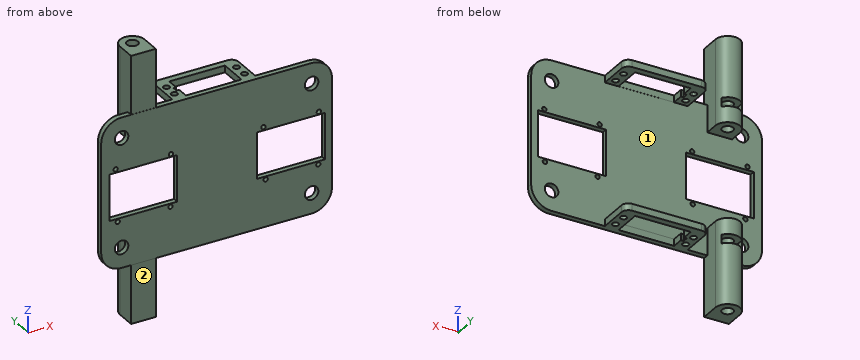
Autodesk Inventor part; units mm, degrees
ref_plane "Work Plane1" through (0, 0, 0) normal (0, 0, -1) x (-1, 0, 0)
ref_plane "YZ Plane" through (0, 0, 0) normal (1, 0, 0) x (0, 1, 0)
ref_plane "XZ Plane" through (0, 0, 0) normal (0, 1, 0) x (-1, 0, 0)
sketch "Sketch1" plane through (0, 0, 0) normal (0, 0, 1) x (1, 0, 0)
  line L0 (-20.5, 0.0342) -> (20.5, 0.0342)
  line L1 (20.5, 0.0342) -> (20.5, 21.0342)
  line L2 (20.5, 21.0342) -> (-20.5, 21.0342)
  line L3 (-20.5, 21.0342) -> (-20.5, 0.0342)
  line L4 (0, -10.9658) -> (0, 38.0342)
  line L5 (20.5, 0.0342) -> (27.5, 0.0342)
  line L6 (20.5, 18.3469) -> (20.5, 0.0342)
  line L7 (20.5, 1.1342) -> (27.5, 1.1342)
  line L8 (27.5, 1.1342) -> (27.5, 19.9342)
  line L9 (27.5, 19.9342) -> (20.5, 19.9342)
  line L10 (20.5, 19.9342) -> (20.5, 1.1342)
  circle A0 centre (25.8, 15.5342) radius 2.3
  circle A1 centre (25.8, 5.5342) radius 2.3
  line L11 (-20.5, 0.0342) -> (-27.5, 0.0342)
  line L12 (-20.5, 1.1342) -> (-27.5, 1.1342)
  line L13 (-27.5, 19.9342) -> (-20.5, 19.9342)
  circle A2 centre (-25.8, 15.5342) radius 2.3
  circle A3 centre (-25.8, 5.5342) radius 2.3
  line L14 (-30.5, 0.0342) -> (-30.5, 31.0342)
  line L15 (30.5, 31.0342) -> (30.5, 0.0342)
  line L16 (-30.5, 26.0342) -> (30.5, 26.0342)
  line L17 (-27.5, 1.1342) -> (-27.5, 13.985)
  line L18 (-27.5, 17.0834) -> (-27.5, 19.9342)
  line L19 (-20.5, 8.5342) -> (-22.5, 8.5342)
  line L20 (-22.5, 8.5342) -> (-22.5, 12.5342)
  line L21 (-22.5, 12.5342) -> (-20.5, 12.5342)
  line L22 (-20.5, 9.5596) -> (-20.5, 7.5596)
  line L23 (-21.9602, 10.5342) -> (-18.6691, 10.5342)
  line L24 (-30.5, 0.0342) -> (-26.5, 0.0342)
  line L25 (-30.5, 0.0342) -> (30.5, 0.0342)
  line L26 (30.5, 0.0342) -> (30.5, -3.9658)
  line L27 (30.5, -3.9658) -> (-30.5, -3.9658)
  line L28 (-30.5, -3.9658) -> (-30.5, 0.0342)
  point P0 (0, 0)
  point P1 (30.5, 0.0342)
  dimension "d0" = 41
  dimension "d4" = 7
  dimension "d5" = 18.8
  dimension "d6" = 1.1
  dimension "d7" = 21
  dimension "d8" = 4.6
  dimension "d9" = 4.6
  dimension "d10" = 5.3
  dimension "d11" = 10
  dimension "d12" = 4.4
  dimension "d13" = 4.4
  dimension "d14" = 10
  dimension "d15" = 5
  dimension "d16" = 2
  dimension "d17" = 4
  dimension "d19" = 4
extrude "Extrusion1" add sketch "Sketch1" along normal blind 5 contours L11 L24 L14 L16 L4 L2 L3 L13 L18 A2 L17 A3 L12 | L0 L4 L27 L28 L24 L11 | L0 L5 L25 L26 L27 L4 | L12 L17 A3 A2 L18 L13 L3 L21 L20 L19 | L1 L7 L8 A1 A0 L9 L2 L4 L16 L15 L25 L5 | L1 L9 L8 A0 A1 L7
sketch "Sketch2" plane through (0, 0, 5) normal (0, 0, 1) x (1, 0, 0)
  line L0 (20.5, 0.0342) -> (-20.5, 0.0342)
  line L1 (20.5, 0.0342) -> (12.9, 0.0342)
  line L2 (12.9, 0.0342) -> (12.9, 10.0342)
  line L3 (12.9, 10.0342) -> (-54.1, 10.0342)
  circle A0 centre (-54.1, 10.0342) radius 4.1
  circle A1 centre (-54.1, 10.0342) radius 9.1
  line L4 (-63.2, 10.0342) -> (-63.2, 0.0342)
  line L5 (-45, 10.0342) -> (-45, 0.0342)
  line L6 (-63.2, 0.0342) -> (-45, 0.0342)
  line L7 (-63.2, 0.0342) -> (-45, 0.0342)
  line L8 (-45, 0.0342) -> (-45, -3.9658)
  line L9 (-45, -3.9658) -> (-63.2, -3.9658)
  line L10 (-63.2, -3.9658) -> (-63.2, 0.0342)
  point P0 (0, 0)
  dimension "d22" = 7.6
  dimension "d23" = 10
  dimension "d24" = 67
  dimension "d25" = 8.2
  dimension "d26" = 5
  dimension "d29" = 4
extrude "Extrusion2" add sketch "Sketch2" along normal blind 43
sketch "Sketch5" plane through (0, 0, 0) normal (0, 1, 0) x (-1, 0, 0)
  line L0 (-20.5, 0) -> (-20.5, 5)
  line L1 (20.5, 0) -> (20.5, 5)
  line L2 (14.7818, 0) -> (56.1092, 0)
  line L3 (56.1092, 0) -> (56.1092, -28.5)
  line L4 (56.1092, -28.5) -> (14.7818, -28.5)
  line L5 (14.7818, -28.5) -> (14.7818, 0)
  line L6 (17.451, -24.4449) -> (17.451, -8.948) construction
  line L7 (17.451, -8.948) -> (25.6459, -8.948) construction
  line L8 (25.6459, -8.948) -> (25.6459, -24.4449) construction
  line L9 (25.6459, -24.4449) -> (17.451, -24.4449) construction
  line L10 (-84.7718, 5) -> (85.2282, 5)
  line L11 (85.2282, 5) -> (85.2282, -50)
  line L12 (85.2282, -50) -> (-84.7718, -50)
  line L13 (-84.7718, -50) -> (-84.7718, 5)
  point P0 (0, 0)
  point P1 (30.5, 5)
  dimension "d30" = 28.5
  dimension "d49" = 55
  dimension "d60" = 170
sketch "Sketch7" plane through (0, 0, 0) normal (0, 1, 0) x (-1, 0, 0)
  point P0 (0, 0)
sketch "Sketch8" plane through (0, 0, 5) normal (0, 0, -1) x (-1, 0, 0)
  line L0 (63.2, 10.0342) -> (63.2, -3.9658)
  arc A0 (63.2, 10.0342) -> (45, 10.0342) centre (54.1, 10.0342) ccw
  line L1 (45, -3.9658) -> (45, 10.0342)
  line L2 (63.2, -3.9658) -> (45, -3.9658)
  circle A1 centre (54.1, 10.0342) radius 4.1
  line L3 (63.2, 10.0342) -> (63.2, -3.9658)
  line L4 (63.2, 0) -> (45, 0)
  point P0 (0, 0)
extrude "Extrusion4" add sketch "Sketch8" along normal blind 20 contours L0 L4 L1 A0
extrude "Extrusion5" add sketch "Sketch5" against normal blind 4 contours L10 L11 L12 L13 | L2 L3 L4 L5
ref_plane "Work Plane1" through (0, 0, 0) normal (0, 0, -1) x (-1, 0, 0)
sketch "Sketch9" plane through (0, 0, 0) normal (0, 0, -1) x (-1, 0, 0)
  line L0 (45, 10.0342) -> (45, 0)
  line L1 (45, 0) -> (63.2, 0)
  line L2 (63.2, 0) -> (63.2, 10.0342)
  arc A0 (63.2, 10.0342) -> (45, 10.0342) centre (54.1, 10.0342) ccw
  circle A1 centre (54.1, 10.0342) radius 4.1
  line L3 (61.6056, 10.0342) -> (57.8528, 3.5342)
  line L4 (57.8528, 3.5342) -> (50.3472, 3.5342)
  line L5 (50.3472, 3.5342) -> (46.5944, 10.0342)
  line L6 (46.5944, 10.0342) -> (50.3472, 16.5342)
  line L7 (50.3472, 16.5342) -> (57.8528, 16.5342)
  line L8 (57.8528, 16.5342) -> (61.6056, 10.0342)
  line L9 (46.5944, 10.0342) -> (46.5944, 15.1797)
  arc A2 (63.2, 10.0342) -> (45, 10.0342) centre (54.1, 10.0342) ccw
  line L10 (61.6056, 10.0342) -> (61.6056, 15.1797)
  point P0 (0, 0)
  dimension "d43" = 13
extrude "Extrusion6" cut sketch "Sketch9" along normal mid plane 6.5 contours A0 L10 L8 L7 L6 L9 | L6 L7 L8 L3 L4 L5
fillet "Fillet2" radius 15 2 edges at (84.7718, -2, 5) (-85.2282, -2, 5)
fillet "Fillet3" radius 5 2 edges at (30.5, 26.0342, 2.5) (-30.5, 26.0342, 2.5)
sketch "Sketch10" plane through (0, 0, 0) normal (0, 1, 0) x (1, 0, 0)
  arc A0 (-85.2282, 10) -> (-70.2282, -5) centre (-70.2282, 10) ccw
  line L0 (-63.2, -5) -> (-63.2, 15)
  line L1 (-45, 15) -> (-63.2, 15)
  line L2 (-45, -5) -> (-45, 15)
  line L3 (-45, -5) -> (-30.5, -5)
  line L4 (-30.5, 0) -> (-30.5, -5)
  line L5 (30.5, 0) -> (-30.5, 0)
  line L6 (30.5, -5) -> (30.5, 0)
  line L7 (30.5, -5) -> (69.7718, -5)
  arc A1 (69.7718, -5) -> (84.7718, 10) centre (69.7718, 10) ccw
  line L8 (84.7718, 10) -> (84.7718, 50)
  line L9 (84.7718, 50) -> (-85.2282, 50)
  line L10 (-85.2282, 50) -> (-85.2282, 10)
  line L11 (-70.2282, -5) -> (-63.2, -5)
  point P0 (0, 0)
hole "Hole1" at (-70.2282, 0, -10) at (69.7718, 0, -10) direction (0, -1, 0) diameter 10 depth 4
mirror "Mirror4" about plane through (-85.2282, 0, -50) normal (0, 0, -1) of "Extrusion1", "Extrusion2", "Extrusion4", "Extrusion5", "Extrusion6", "Fillet2", "Fillet3", "Hole1"
sketch "Sketch11" plane through (0, 0, 0) normal (0, 1, 0) x (1, 0, 0)
  circle A0 centre (69.7718, 90) radius 5
  circle A1 centre (69.7718, 10) radius 5
  arc A2 (-70.2282, 105) -> (-85.2282, 90) centre (-70.2282, 90) ccw
  line L0 (-85.2282, 90) -> (-85.2282, 10)
  arc A3 (-85.2282, 10) -> (-70.2282, -5) centre (-70.2282, 10) ccw
  line L1 (-63.2, -5) -> (-63.2, 15)
  line L2 (-45, 15) -> (-63.2, 15)
  line L3 (-45, -5) -> (-45, 15)
  line L4 (-45, -5) -> (-30.5, -5)
  line L5 (-30.5, 0) -> (-30.5, -5)
  line L6 (30.5, 0) -> (-30.5, 0)
  line L7 (30.5, -5) -> (30.5, 0)
  line L8 (30.5, -5) -> (69.7718, -5)
  arc A4 (69.7718, -5) -> (84.7718, 10) centre (69.7718, 10) ccw
  line L9 (84.7718, 10) -> (84.7718, 90)
  arc A5 (84.7718, 90) -> (69.7718, 105) centre (69.7718, 90) ccw
  line L10 (30.5, 105) -> (69.7718, 105)
  line L11 (30.5, 105) -> (30.5, 100)
  line L12 (30.5, 100) -> (-30.5, 100)
  line L13 (-30.5, 100) -> (-30.5, 105)
  line L14 (-45, 105) -> (-30.5, 105)
  line L15 (-45, 105) -> (-45, 85)
  line L16 (-45, 85) -> (-63.2, 85)
  line L17 (-63.2, 105) -> (-63.2, 85)
  line L18 (20.5, 100) -> (-20.5, 100)
  line L19 (20.5, 100) -> (20.5, 105)
  line L20 (20.5, 105) -> (-20.5, 105)
  line L21 (-20.5, 100) -> (-20.5, 105)
  line L22 (-20.5, 100) -> (20.5, 100)
  line L23 (20.5, 100) -> (20.5, 71.5)
  line L24 (20.5, 71.5) -> (-20.5, 71.5)
  line L25 (-20.5, 71.5) -> (-20.5, 100)
  line L26 (74.1747, 78.4479) -> (24.1747, 78.4479)
  line L27 (24.1747, 78.4479) -> (24.1747, 28.4479)
  line L28 (24.1747, 28.4479) -> (74.1747, 28.4479)
  line L29 (74.1747, 28.4479) -> (74.1747, 78.4479)
  line L30 (0, 73.183) -> (0, 43.8378)
  line L31 (-78.2096, 79.1815) -> (-28.2096, 79.1815)
  line L32 (-28.2096, 79.1815) -> (-28.2096, 29.1815)
  line L33 (-28.2096, 29.1815) -> (-78.2096, 29.1815)
  line L34 (-78.2096, 29.1815) -> (-78.2096, 79.1815)
  circle A6 centre (-70.2282, 90) radius 5
  line L35 (-70.2282, 105) -> (-63.2, 105)
  line L36 (-70.2282, -5) -> (-63.2, -5)
  circle A7 centre (-70.2282, 10) radius 5
  point P0 (0, 0)
  dimension "d57" = 28.5
  dimension "d58" = 50
  dimension "d59" = 50
sketch "Sketch12" plane through (0, 0, 0) normal (0, 1, 0) x (1, 0, 0)
  line L0 (-79.2036, 26.0949) -> (-29.2036, 26.0949)
  line L1 (-29.2036, 26.0949) -> (-29.2036, 76.0949)
  line L2 (-29.2036, 76.0949) -> (-79.2036, 76.0949)
  line L3 (-79.2036, 76.0949) -> (-79.2036, 26.0949)
  circle A0 centre (-74.6036, 31.6949) radius 1.6
  line L4 (-85.2282, 90) -> (-85.2282, 10)
  circle A1 centre (-33.8036, 32.0949) radius 1.6
  circle A2 centre (-34.2036, 70.4949) radius 1.6
  line L5 (-79.2036, 34.2067) -> (-29.2036, 34.2067)
  line L6 (-29.2036, 34.2067) -> (-29.2036, 68.2067)
  line L7 (-29.2036, 68.2067) -> (-79.2036, 68.2067)
  line L8 (-79.2036, 68.2067) -> (-79.2036, 34.2067)
  circle A3 centre (-73.0036, 70.4949) radius 1.6
  line L9 (29.7223, 26.0949) -> (79.7223, 26.0949)
  line L10 (79.7223, 26.0949) -> (79.7223, 76.0949)
  line L11 (79.7223, 76.0949) -> (29.7223, 76.0949)
  line L12 (29.7223, 76.0949) -> (29.7223, 26.0949)
  circle A4 centre (34.3223, 31.6949) radius 1.6
  circle A5 centre (75.1223, 32.0949) radius 1.6
  circle A6 centre (74.7223, 70.4949) radius 1.6
  line L13 (29.7223, 34.2067) -> (79.7223, 34.2067)
  line L14 (79.7223, 34.2067) -> (79.7223, 68.2067)
  line L15 (79.7223, 68.2067) -> (29.7223, 68.2067)
  line L16 (29.7223, 68.2067) -> (29.7223, 34.2067)
  circle A7 centre (35.9223, 70.4949) radius 1.6
  point P0 (0, 0)
  dimension "d67" = 50
  dimension "d68" = 50
  dimension "d69" = 3.2
  dimension "d70" = 4.6
  dimension "d71" = 10.6246
  dimension "d72" = 5.6
  dimension "d73" = 3.2
  dimension "d74" = 4.6
  dimension "d75" = 3.2
  dimension "d76" = 5.6
  dimension "d88" = 34
  dimension "d89" = 3.2
  dimension "d90" = 50
  dimension "d91" = 50
  dimension "d92" = 3.2
  dimension "d93" = 4.6
  dimension "d94" = 5.6
  dimension "d95" = 3.2
  dimension "d96" = 4.6
  dimension "d97" = 3.2
  dimension "d98" = 5.6
  dimension "d99" = 34
  dimension "d100" = 3.2
extrude "Extrusion7" cut sketch "Sketch12" against normal up to next contours L3 L7 L1 L5 | A0 | A1 | A2 | A3 | L12 L15 L10 L13 | A4 | A5 | A6 | A7
equation "\"d6\" = -0.5 * d5 + 0.5 * d7"
equation "\"d12\" = d13"
equation "\"d73\" = d69"
equation "\"d74\" = d70"
equation "\"d75\" = d69"
equation "\"d76\" = d72"
equation "\"d89\" = d69"
equation "\"d95\" = d92"
equation "\"d96\" = d93"
equation "\"d97\" = d92"
equation "\"d98\" = d94"
equation "\"d100\" = d92"
properties part number "Base" material "PLA"
The listing builds one solid part. Answer for the finished solid, in the listing's coordinates (mm). Face numbers are marked on the shaded views. Give positions to 0.01 mm unless a question says otherwise; leave off trailing zeros. Order: outer loops, then holes, each group sorted by start corner. A loop starts at its lowest first (then second) coordinate and runs counter-clockwise, first axis right, second up. Notation, with made-up numbers: (78.5, 77) - (135.5, 77) arc R29 ccw to (135.5, 99) - close; hole circle Ø9 at (61.5, -24.75). An arc over 180 degrees is marked (long way). Answer in a Markdown table with one row per item. Add a question column.
Q1. The part is cut by section B-B (x = -13.5). Give the number of separate pieces and of enclosed holes in the cut face, then the cut area to 3 significant figures.
Q2. Find the intervals of material crossed by line 1 along Z through (x, y) = (-52.5, 15); line 2 along Y through (x, z) = (25.8, 1.3); line 3 along X through (y, z) = (10, 2), in increasing order. Write a range as [from, to].
Q3. The part is cut by section A-A (z = -65). Determine the outline of the cut face in (x, y), then the cut area to 3 significant figures.
Q4. For a pull along Z with two mould halves and no side action, classify the marked faces 1 and 2 as released by +Z, released by -Z, zero draft, split by the parting line, or undercut.
Q5. Given P1, Ø11, axis at y = 1, z = -129.5, coming from the +X side; P2, Ø5, axis at x = -33.8, z = -32.09, coming from the -Y side; P3, Ø4, axis at x = 35.92, z = -70.49, coming from the +Y side; P4, Ø2.5, axis at x = -73, z = -70.49, coming from the +Y side, each flat-ended and moving along its own axis, determine where each tip first touches the part or whether it passes through.
Determined:
| question | item | result |
|---|---|---|
| 1 | separate pieces | 3 |
| 1 | enclosed holes | 0 |
| 1 | area | 490 mm² |
| 2 | line 1 | z = [-148, -103.25], [-96.75, -85], [-15, -3.25], [3.25, 48] |
| 2 | line 2 | y = [-4, 3.23], [7.83, 13.23], [17.83, 26.03] |
| 2 | line 3 | x = [-63.2, -61.59], [-46.61, -45], [-30.5, -22.5], [20.5, 30.5] |
| 3 | outline | (-85.23, -4) - (-79.2, -4) - (-79.2, 0) - (-85.23, 0) - close; (-29.2, -4) - (29.72, -4) - (29.72, 0) - (-29.2, 0) - close; (79.72, -4) - (84.77, -4) - (84.77, 0) - (79.72, 0) - close |
| 3 | area | 280 mm² |
| 4 | face 1 | undercut |
| 4 | face 2 | zero draft |
| 5 | P1 | stops at x = -45 |
| 5 | P2 | stops at y = -4 |
| 5 | P3 | stops at y = 0 |
| 5 | P4 | passes through |
